Check sheet for the modelled part. Datum: model origin and axes. Units: mm. A direction names the side the tool comes from. Round coordinates to 2 decimals unless told otherwise and drop trailing zeros. Order: outer loops, then holes, each group sorted by start corner. A loop starts at its lowest first (then second) coordinate and runs counter-clockwise, first axis right, second up.
Solid Edge part; units mm, degrees
sketch "Sketch1" plane through (0, 0, 0) normal (0, -1, 0) x (1, 0, 0)
  line L0 (0, 6) -> (4.4, 6)
  line L1 (4.4, 6) -> (5, 5.4)
  line L2 (5, 5.4) -> (5, 0)
  line L3 (5, 0) -> (3, 0)
  line L4 (3, 0) -> (3, -34)
  line L5 (3, -34) -> (2, -35)
  line L6 (2, -35) -> (0, -35)
  line L7 (0, -35) -> (0, 6)
  dimension "D1" = 3
  dimension "D2" = 4.4
revolve "RevolvedProtrusion1" add sketch "Sketch1" angle 360 about axis through (0, 0, 54) along (0, 0, -1)
sketch "Sketch2" plane through (0, 0, 6) normal (0, 0, 1) x (0, 1, 0)
  line L0 (-2.8868, 0) -> (-1.4434, 2.5)
  line L1 (-1.4434, 2.5) -> (1.4434, 2.5)
  line L2 (1.4434, 2.5) -> (2.8868, 0)
  line L3 (2.8868, 0) -> (1.4434, -2.5)
  line L4 (1.4434, -2.5) -> (-1.4434, -2.5)
  line L5 (-1.4434, -2.5) -> (-2.8868, 0)
extrude "Cutout1" cut sketch "Sketch2" against normal blind 3
sketch "Sketch3" plane through (0, 0, 0) normal (0, -1, 0) x (1, 0, 0)
  line L0 (3, -11) -> (2.5, -11)
  line L1 (2.5, -11) -> (2.5, -11.05)
  line L2 (2.5, -11.05) -> (3, -11.05)
revolve "RevolvedCutout1" cut sketch "Sketch3" angle 360 about axis through (0, 0, 54) along (0, 0, -1) material side at (2.75, 0, -11.05)
cosmetic_thread "Thread1"
properties material "Steel"
Item 1: Scan lines: line 1 along Z through (x, y) = (0, 1); line 2 along Z through (x, y) = (-4, -1.75); line 3 along Y through (x, z) = (0, -32.5). Record each from-to range of solid material in increasing order.
Answer:
line 1: z = -35 to 3
line 2: z = 0 to 6
line 3: y = -3 to 3
Item 2: Access from +Z, -Z, +X, -X, +Y, -Y to the whole of each face (thin tool, end or side, straight path). Record for faces 1 (the cylindrical face through (-1.08, 4.88, 2.66)), 2 (the cylindrical face through (-3, 0, -6)), 3 (the flat face through (-1.233, -2.175, 4.521)).
Answer:
face 1: +Z, -Z
face 2: -Z
face 3: +Z
Item 3: Go/stop test with flat-tipped pins: P1, Ø5, axis at y = -4, z = -3, coming from the -X side; P2, Ø3, axis at x = -1.5, z = -17, coming from the +Y side; P3, Ø1.5, axis at y = 3, z = -22, coming from the +X side. Record where each tip stops, or that it passes through.
Answer:
P1: stops at x = -2.6
P2: stops at y = 3
P3: stops at x = 1.98
Item 4: Release check for a two-part mould opening along Y. For faces 4 (the flat face through (1.267, -2.155, 4.521)), 5 (the cylindrical face through (-3, 0, -23)), 6 (the flat face through (0, 0, 3)), 7 (the flat face through (3.3, -0.1, 0)) record: released by +Y, released by -Y, zero draft, split by the parting line, or undercut.
Answer:
face 4: undercut
face 5: split by the parting line
face 6: undercut
face 7: zero draft
Item 5: Sectioned sample at C-C (z = -19.5). Record the cut outline in (x, y).
Answer:
outline: circle Ø6 at (0, 0)
Item 6: Sectioned sample at B-B (z = 2). Record the cut outline in (x, y).
Answer:
outline: circle Ø10 at (0, 0)
Item 7: Sectioned sample at A-A (y = 0). Record the cut outline in (x, z), and give its area (3 significant figures).
Answer:
outline: (-5, 0) - (-3, 0) - (-3, -11) - (-2.5, -11) - (-2.5, -11.05) - (-3, -11.05) - (-3, -34) - (-2, -35) - (2, -35) - (3, -34) - (3, -11.05) - (2.5, -11.05) - (2.5, -11) - (3, -11) - (3, 0) - (5, 0) - (5, 5.4) - (4.4, 6) - (2.5, 6) - (2.5, 3) - (-2.5, 3) - (-2.5, 6) - (-4.4, 6) - (-5, 5.4) - close
area: 254 mm2
